Could you check a few things on this model? Use its own coordinates, in mm. A direction names the side the tool comes from. Round coordinates to 2 decimals unless told otherwise and drop trailing zeros. Write each loop counter-clockwise with the first axis right and the second up, starting at its lowest first coordinate (ties: lowest second). Pieces come first, ordered by that corner, then holes.
```python
from build123d import *

# Parameters (mm, degrees)
BOSS_EXTRUDE1_DEPTH = 6.5
BOSS_EXTRUDE2_DEPTH = 6.5
SKETCH2_R           = 1.6
BOSS_EXTRUDE3_DEPTH = 55


with BuildPart() as part:
    # Sketch1 → Boss-Extrude1 (new body)
    with BuildSketch(Plane.XY):
        Polygon((9.277156847, 35.75), (13.377156847, 35.75), (13.377156847, 27.05), (19.777156847, 27.05), (19.777156847, 35.75), (24.077156847, 35.75), (24.077156847, 40.25), (9.277156847, 40.25), align=None)
    extrude(amount=BOSS_EXTRUDE1_DEPTH)



with BuildPart() as body_2:
    # Sketch1<6> → Boss-Extrude2 (new body)
    with BuildSketch(Plane.XY):
        Polygon((8.177156847, -42.25), (24.977156847, -42.25), (24.977156847, -25.85), (19.577156847, -25.85), (19.577156847, -22.85), (13.577156847, -22.85), (13.577156847, -25.85), (8.177156847, -25.85), align=None)
    extrude(amount=BOSS_EXTRUDE2_DEPTH)


with BuildPart() as part_1:
    add(part.part)

    add(body_2.part)  # Boss-Extrude3 merges body 2
    # Sketch2 → Boss-Extrude3 (add)
    with BuildSketch(Plane.XZ.offset(-27.05)):
        with Locations((16.577156847, 3.25)):
            Circle(SKETCH2_R)
    extrude(amount=BOSS_EXTRUDE3_DEPTH)


solid = part_1.part
```
Q1. We'd pull the mould along Y, two halves only. Please class faces 1 (the flat face through (16, -32, 6.5)), 2 (the flat face through (16, -42.25, 3)), 3 (the flat face through (11, 35.75, 3)): pulls with the +Y half, pulls with the -Y half, needs draft (parallel to the pull), parting line crosses it, or undercut.
Q2. If I drill on L1, parallel to Y at x = 12, z = 2; L2, parallel to Y at x = 16, z = 5.5; L3, parallel to X at y = 29, z = 6.25, over which ranges is the centre line in solid material (lowest first)?
Q3. Imagine slicing it at A-A, the plane x = 22.25. Write out the boundary of the cut face in (y, z), then the cut area to 3 significant figures.
Q4. Imagine slicing it at B-B, the plane z = 3.25. Write out the boundary of the cut face in (x, y).
Q5. I'm going to push flat-ended pins straight in: pin 1 Ø2 at (y, z) = (23.5, 1.5) entering from +X; pin 2 Ø3.5 at (y, z) = (-24, 2.5) entering from +X; pin 3 Ø0.9 at (y, z) = (-24.5, 3.5) entering from -X. Where does each tip first touch, or does it pass through?
Q6. Imagine slicing it at C-C, the plane y = 23.5. Write out the boundary of the cut face in (x, z).
Q7. On a 3-axis mill with a long thin cutter (end or side, diameter ignored), from which of +Z, -Z, +X, -X, +Y, -Y can I reach the whole of each face in a straight line? I mean faces 4 (the flat face through (24.077, 38, 3)), 5 (the cylindrical face through (14.98, 2.45, 3.32)), 6 (the flat face through (19.577, -24, 3)). Say none if no direction works.
Results found:
1. face 1: needs draft
1. face 2: pulls with the -Y half
1. face 3: undercut
2. L1: y = -42.25 to -25.85, 35.75 to 40.25
2. L2: y = -42.25 to -22.85, 27.05 to 40.25
2. L3: x = 13.38 to 19.78
3. outline: (-42.25, 0) - (-25.85, 0) - (-25.85, 6.5) - (-42.25, 6.5) - close; (35.75, 0) - (40.25, 0) - (40.25, 6.5) - (35.75, 6.5) - close
3. area: 136 mm2
4. outline: (8.18, -42.25) - (24.98, -42.25) - (24.98, -25.85) - (19.58, -25.85) - (19.58, -22.85) - (18.18, -22.85) - (18.18, 27.05) - (19.78, 27.05) - (19.78, 35.75) - (24.08, 35.75) - (24.08, 40.25) - (9.28, 40.25) - (9.28, 35.75) - (13.38, 35.75) - (13.38, 27.05) - (14.98, 27.05) - (14.98, -22.85) - (13.58, -22.85) - (13.58, -25.85) - (8.18, -25.85) - close
5. pin 1: stops at x = 17.99
5. pin 2: stops at x = 19.58
5. pin 3: stops at x = 13.58
6. outline: circle Ø3.2 at (16.58, 3.25)
7. face 4: +Z, -Z, +X, +Y
7. face 5: none
7. face 6: +Z, -Z, +X
